Design review of the part built by this model. Coordinates are the model's own, in mm. A direction names the side the tool comes from. Round coordinates to 2 decimals unless told otherwise and drop trailing zeros. Loops run counter-clockwise (first coordinate to the right, second up) from the corner with the lowest first, then second, coordinate; pieces in that order, holes last. Notation, with made-up numbers: (-25.5, 84.25) -> (-7.5, 84.25) arc R20 ccw to (-7.5, 117.25) -> close; hole circle Ø3 at (44.5, -22.75). An arc over 180 degrees is marked (long way). Write each question's results on one line, items separated by ' | '. Start each with the question number.
Autodesk Inventor part; units mm, degrees
ref_plane "YZ Plane" through (0, 0, 0) normal (1, 0, 0) x (0, 1, 0)
ref_plane "XZ Plane" through (0, 0, 0) normal (0, 1, 0) x (-1, 0, 0)
ref_plane "XY Plane" through (0, 0, 0) normal (0, 0, 1) x (1, 0, 0)
sketch "Sketch6" plane through (0, 0, 0) normal (1, 0, 0) x (0, 1, 0)
  line L0 (-25.4, 31.75) -> (-25.4, -31.75)
  line L1 (-25.4, -31.75) -> (0, -31.75)
  line L2 (0, -31.75) -> (0, 31.75)
  line L3 (0, 31.75) -> (-25.4, 31.75)
  line L4 (-25.4, 31.75) -> (0, -31.75) construction
  line L5 (-25.4, -31.75) -> (0, 31.75) construction
  line L6 (0, 31.75) -> (0, -31.75)
  line L7 (0, -31.75) -> (50.8, -31.75)
  line L8 (50.8, -31.75) -> (50.8, 31.75)
  line L9 (50.8, 31.75) -> (0, 31.75)
  line L10 (0, 31.75) -> (50.8, -31.75) construction
  line L11 (0, -31.75) -> (50.8, 31.75) construction
  circle A0 centre (39.6875, -20.6375) radius 4.7625
  point P0 (0, 0)
  point P1 (-12.7, 0)
  point P2 (25.4, 0)
  dimension "d12" = 12.7
  dimension "d13" = 25.4
  dimension "d14" = 50.8
  dimension "d15" = 25.4
  dimension "d16" = 9.525
  dimension "d17" = 11.1125
  dimension "d18" = 11.1125
  dimension "d24" = 63.5
extrude "Extrusion3" add sketch "Sketch6" along normal mid plane 19.05
sketch "Sketch7" plane through (-9.525, -25.4, 31.75) normal (0, 0, 1) x (1, 0, 0)
  line L0 (9.525, 25.4) -> (9.525, 0) construction
  line L1 (0, 0) -> (19.05, 0) construction
  line L2 (4.7625, 0) -> (14.2875, 0)
  line L3 (14.2875, 0) -> (14.2875, 25.4)
  line L4 (14.2875, 25.4) -> (4.7625, 25.4)
  line L5 (4.7625, 25.4) -> (4.7625, 0)
  line L6 (4.7625, 0) -> (14.2875, 25.4) construction
  line L7 (14.2875, 0) -> (4.7625, 25.4) construction
  point P0 (9.525, 12.7)
  dimension "d21" = 9.525
extrude "Extrusion4" cut sketch "Sketch7" against normal through all
sketch "Sketch8" plane through (9.525, 0, 0) normal (1, 0, 0) x (0, 0, -1)
  line L0 (31.75, -25.4) -> (31.75, 0)
  line L1 (-31.75, -25.4) -> (31.75, -25.4)
  line L2 (-31.75, 0) -> (-31.75, -25.4)
  line L3 (-31.75, 0) -> (31.75, 0)
  line L4 (-292.1, -85.725) -> (-292.1, -12.7)
  arc A0 (-292.1, -85.725) -> (-279.4, -98.425) centre (-279.4, -85.725) ccw
  line L5 (222.25, -98.425) -> (-279.4, -98.425)
  arc A1 (222.25, -98.425) -> (234.95, -85.725) centre (222.25, -85.725) ccw
  line L6 (234.95, -81.1401) -> (234.95, -85.725)
  arc A2 (234.95, -81.1401) -> (231.6119, -72.5584) centre (222.25, -81.1401) ccw
  line L7 (231.6119, -72.5584) -> (168.8751, -4.1183)
  arc A3 (168.8751, -4.1183) -> (159.5132, 0) centre (159.5132, -12.7) ccw
  line L8 (159.5132, 0) -> (-279.4, 0)
  arc A4 (-279.4, 0) -> (-292.1, -12.7) centre (-279.4, -12.7) ccw
  circle A5 centre (215.9, -79.375) radius 4.826
  circle A6 centre (-241.3, -79.375) radius 4.826
  circle A7 centre (200.025, -79.375) radius 4.826
  circle A8 centre (182.9995, -40.6685) radius 3.3782
  circle A9 centre (165.1, -85.725) radius 3.3782
  line L9 (-236.5375, -55.8157) -> (-236.5375, -25.4)
  arc A10 (-233.3625, -22.225) -> (-236.5375, -25.4) centre (-233.3625, -25.4) ccw
  line L10 (-233.3625, -22.225) -> (-210.2431, -22.225)
  arc A11 (-207.7154, -27.3213) -> (-210.2431, -22.225) centre (-210.2431, -25.4) ccw
  line L11 (-207.7154, -27.3213) -> (-230.8348, -57.737)
  arc A12 (-236.5375, -55.8157) -> (-230.8348, -57.737) centre (-233.3625, -55.8157) ccw
  line L12 (-229.0307, -71.1037) -> (-201.0846, -34.338)
  arc A13 (-195.3819, -36.2593) -> (-201.0846, -34.338) centre (-198.5569, -36.2593) ccw
  line L13 (-195.3819, -36.2593) -> (-195.3819, -73.025)
  arc A14 (-198.5569, -76.2) -> (-195.3819, -73.025) centre (-198.5569, -73.025) ccw
  line L14 (-198.5569, -76.2) -> (-226.503, -76.2)
  arc A15 (-229.0307, -71.1037) -> (-226.503, -76.2) centre (-226.503, -73.025) ccw
  line L15 (-73.119, -73.025) -> (-73.119, -34.8804)
  arc A16 (-67.6008, -32.738) -> (-73.119, -34.8804) centre (-69.944, -34.8804) ccw
  line L16 (-67.6008, -32.738) -> (-32.724, -70.8826)
  arc A17 (-35.0672, -76.2) -> (-32.724, -70.8826) centre (-35.0672, -73.025) ccw
  line L17 (-35.0672, -76.2) -> (-69.944, -76.2)
  arc A18 (-73.119, -73.025) -> (-69.944, -76.2) centre (-69.944, -73.025) ccw
  line L18 (34.0449, -27.5424) -> (-2.4193, -67.4233)
  arc A19 (-7.9375, -65.2808) -> (-2.4193, -67.4233) centre (-4.7625, -65.2808) ccw
  line L19 (-7.9375, -65.2808) -> (-7.9375, -25.4)
  arc A20 (-4.7625, -22.225) -> (-7.9375, -25.4) centre (-4.7625, -25.4) ccw
  line L20 (-4.7625, -22.225) -> (31.7017, -22.225)
  arc A21 (34.0449, -27.5424) -> (31.7017, -22.225) centre (31.7017, -25.4) ccw
  line L21 (-22.9807, -67.4233) -> (-59.4449, -27.5424)
  arc A22 (-57.1017, -22.225) -> (-59.4449, -27.5424) centre (-57.1017, -25.4) ccw
  line L22 (-57.1017, -22.225) -> (-20.6375, -22.225)
  arc A23 (-17.4625, -25.4) -> (-20.6375, -22.225) centre (-20.6375, -25.4) ccw
  line L23 (-17.4625, -25.4) -> (-17.4625, -65.2808)
  arc A24 (-22.9807, -67.4233) -> (-17.4625, -65.2808) centre (-20.6375, -65.2808) ccw
  line L24 (47.719, -34.8804) -> (47.719, -73.025)
  arc A25 (44.544, -76.2) -> (47.719, -73.025) centre (44.544, -73.025) ccw
  line L25 (44.544, -76.2) -> (9.6672, -76.2)
  arc A26 (7.324, -70.8826) -> (9.6672, -76.2) centre (9.6672, -73.025) ccw
  line L26 (7.324, -70.8826) -> (42.2008, -32.738)
  arc A27 (47.719, -34.8804) -> (42.2008, -32.738) centre (44.544, -34.8804) ccw
  line L27 (84.1375, -25.4) -> (84.1375, -73.025)
  arc A28 (80.9625, -76.2) -> (84.1375, -73.025) centre (80.9625, -73.025) ccw
  line L28 (80.9625, -76.2) -> (60.419, -76.2)
  arc A29 (57.244, -73.025) -> (60.419, -76.2) centre (60.419, -73.025) ccw
  line L29 (57.244, -73.025) -> (57.244, -25.4)
  arc A30 (60.419, -22.225) -> (57.244, -25.4) centre (60.419, -25.4) ccw
  line L30 (60.419, -22.225) -> (80.9625, -22.225)
  arc A31 (84.1375, -25.4) -> (80.9625, -22.225) centre (80.9625, -25.4) ccw
  line L31 (142.875, -69.85) -> (142.875, -29.1831)
  arc A32 (148.4044, -27.053) -> (142.875, -29.1831) centre (146.05, -29.1831) ccw
  line L32 (148.4044, -27.053) -> (188.0708, -70.8949)
  arc A33 (185.7165, -76.2) -> (188.0708, -70.8949) centre (185.7165, -73.025) ccw
  line L33 (185.7165, -76.2) -> (149.225, -76.2)
  arc A34 (142.875, -69.85) -> (149.225, -76.2) centre (149.225, -69.85) ccw
  circle A35 centre (-173.7792, -57.6072) radius 5.5626
  circle A36 centre (-96.3092, -32.2072) radius 5.5626
  circle A37 centre (-173.7792, -32.2072) radius 5.5626
  circle A38 centre (-96.3092, -57.6072) radius 5.5626
  circle A39 centre (101.6, -28.575) radius 2.5527
  circle A40 centre (111.125, -19.05) radius 2.5527
  circle A41 centre (120.65, -9.525) radius 2.5527
  circle A42 centre (101.6, -88.9) radius 2.5527
  circle A43 centre (120.65, -69.85) radius 2.5527
  circle A44 centre (111.125, -79.375) radius 2.5527
  circle A45 centre (-266.7, -12.7) radius 3.3782
  circle A46 centre (-266.7, -85.725) radius 3.3782
  circle A47 centre (-241.3, -12.7) radius 3.3782
  circle A48 centre (-215.9, -12.7) radius 3.3782
  circle A49 centre (-215.9, -85.725) radius 3.3782
  circle A50 centre (-190.5, -12.7) radius 3.3782
  circle A51 centre (-165.1, -12.7) radius 3.3782
  circle A52 centre (-165.1, -85.725) radius 3.3782
  circle A53 centre (-139.7, -12.7) radius 3.3782
  circle A54 centre (-139.7, -85.725) radius 3.3782
  circle A55 centre (-114.3, -12.7) radius 3.3782
  circle A56 centre (-114.3, -85.725) radius 3.3782
  circle A57 centre (-88.9, -12.7) radius 3.3782
  circle A58 centre (-63.5, -12.7) radius 3.3782
  circle A59 centre (-63.5, -85.725) radius 3.3782
  circle A60 centre (-38.1, -12.7) radius 3.3782
  circle A61 centre (-38.1, -85.725) radius 3.3782
  circle A62 centre (-12.7, -12.7) radius 3.3782
  circle A63 centre (12.7, -12.7) radius 3.3782
  circle A64 centre (12.7, -85.725) radius 3.3782
  circle A65 centre (38.1, -12.7) radius 3.3782
  circle A66 centre (38.1, -85.725) radius 3.3782
  circle A67 centre (63.5, -12.7) radius 3.3782
  circle A68 centre (63.5, -85.725) radius 3.3782
  circle A69 centre (88.9, -12.7) radius 3.3782
  circle A70 centre (88.9, -85.725) radius 3.3782
  circle A71 centre (139.7, -12.7) radius 3.3782
  circle A72 centre (139.7, -85.725) radius 3.3782
  circle A73 centre (161.925, -15.875) radius 4.953
  circle A74 centre (-190.6194, -90.5002) radius 3.3528
  circle A75 centre (-79.469, -90.5002) radius 3.3528
  circle A76 centre (-135.0442, -60.325) radius 14.2812
  circle A77 centre (-12.7, -83.185) radius 4.826
  circle A78 centre (-12.7, -12.7) radius 3.3782
  circle A79 centre (12.7, -12.7) radius 3.3782
  point P0 (0, 0)
extrude "Extrusion5" cut sketch "Sketch8" against normal through all contours A62 | A63
properties part number "WideSupportForLift" material "Aluminum 6061"
1) Insertion check: pin 1 (4 mm diameter, centred on y = -12.7, z = 12.7, fed in from +X); pin 2 (10.5 mm diameter, centred on x = 1, z = -15, fed in from -Y); pin 3 (4 mm diameter, centred on x = -0.5, z = -20, fed in from -Y). Each pin has a flat end and moves straight along its axis. Give the tip position at first contact, or say it passes through.
2) To check wall thickness, follow line 1 (X direction, y = -11, z = 7) (1 decimal); line 2 (Y direction, x = -8, z = -11.5); line 3 (Y direction, x = 8.55, z = -12.7). State the ranges of each line that lie inside material, in increasing order. Write a range as from..to.
3) The part is to be moulded in two halves that separate along X. For faces 1 (the face through (9.525, 12, 0)), 2 (the face through (-7, -25.4, 0)), 3 (the face through (0, 0, 0)), say which applies: +X half, -X half, draft (parallel to the pull), parting line (faces both ways), or undercut.
4) Take a section at B-B (z = -12.7). Write out the cut boundary in (x, y) (1 decimal), plus the area to 3 significant figures.
5) Take a section at A-A (y = -12.7). State how many separate pieces and enclosed holes the cut face has, plus the area to 3 significant figures.
6) For faces 4 (the face through (-4.762, -13, 0)), 5 (the face through (0, 50.8, 0)), list the 3-axis set-ups (+Z, -Z, +X, -X, +Y, -Y) from which the entire face can be reached by the end or side of a thin tool; tool diameter is ignored.
7) Take a section at D-D (z = 7). Write out the cut boundary in (x, y) (1 decimal), plus the area to 3 significant figures.
Geometry check:
1) pin 1: passes through | pin 2: stops at y = -25.4 | pin 3: stops at y = 0
2) line 1: x = -9.5..-4.8, 4.8..9.5 | line 2: y = -25.4..-15.86, -9.54..50.8 | line 3: y = -25.4..-16.08, -9.32..50.8
3) face 1: +X half | face 2: draft | face 3: undercut
4) outline: (-9.5, -25.4) -> (-4.8, -25.4) -> (-4.8, -16.1) -> (-9.5, -16.1) -> close; (-9.5, -9.3) -> (-4.8, -9.3) -> (-4.8, 0) -> (4.8, 0) -> (4.8, -9.3) -> (9.5, -9.3) -> (9.5, 50.8) -> (-9.5, 50.8) -> close; (4.8, -25.4) -> (9.5, -25.4) -> (9.5, -16.1) -> (4.8, -16.1) -> close | area: 1,150 mm^2
5) separate pieces: 6 | enclosed holes: 0 | area: 476 mm^2
6) face 4: +Z, -Z, -Y | face 5: +Z, -Z, +X, -X, +Y
7) outline: (-9.5, -25.4) -> (-4.8, -25.4) -> (-4.8, 0) -> (4.8, 0) -> (4.8, -25.4) -> (9.5, -25.4) -> (9.5, 50.8) -> (-9.5, 50.8) -> close | area: 1,210 mm^2
